from build123d import *

# Parameters (mm, degrees)
SKETCH044_R             = 6.3
SKETCH044_R_2           = 4.2
PAD022_DEPTH            = 0.4
SKETCH049_R             = 5
SKETCH049_R_2           = 4.2
PAD027_DEPTH            = 1.2
PAD037_DEPTH            = 0.2
POLARPATTERN_COUNT      = 6
FILLET002_R             = 0.4
BODY009_PLACEMENT_ANGLE = 153


with BuildPart() as part:
    # Sketch044 → Pad022 (new body)
    with BuildSketch(Plane.XY):
        with Locations((1, 0)):
            Circle(SKETCH044_R)
        Circle(SKETCH044_R_2, mode=Mode.SUBTRACT)
    extrude(amount=PAD022_DEPTH)

    # Sketch049 (on Face4 of Pad022) → Pad027 (join)
    with BuildSketch(Plane.XY.offset(0.4)):
        Circle(SKETCH049_R)
        Circle(SKETCH049_R_2, mode=Mode.SUBTRACT)
    extrude(amount=PAD027_DEPTH)

    # Sketch074 (on Face2 of Pad027) → Pad037 (join)
    with BuildSketch(Plane(origin=(0, 0, 0), x_dir=(1, 0, 0), z_dir=(0, 0, -1))):
        with BuildLine():
            ThreePointArc((3.95, -1.4274102424), (4.2, 0), (3.95, 1.4274102424))
            Line((3.95, 1.4274102424), (3.95, -1.4274102424))
        make_face()
    pad037 = extrude(amount=-PAD037_DEPTH)

    # PolarPattern: Pad037 ×6 about axis
    polarpattern_axis = Axis((0, 0, 0), (0, 0, -1))
    for i in range(1, POLARPATTERN_COUNT):
        add(pad037.rotate(polarpattern_axis, i * 360 / POLARPATTERN_COUNT))

    # Fillet002
    fillet002_edges = [part.edges().sort_by_distance(p)[0] for p in [
        (-4.2, 0, 1.6),
    ]]
    fillet(fillet002_edges, radius=FILLET002_R)


with BuildPart() as part_1:
    # Body009 placement: moved
    add(part.part.moved(Location((0, 0, 4))).rotate(Axis((0, 0, 4), (0, 0, 1)), BODY009_PLACEMENT_ANGLE))


solid = part_1.part
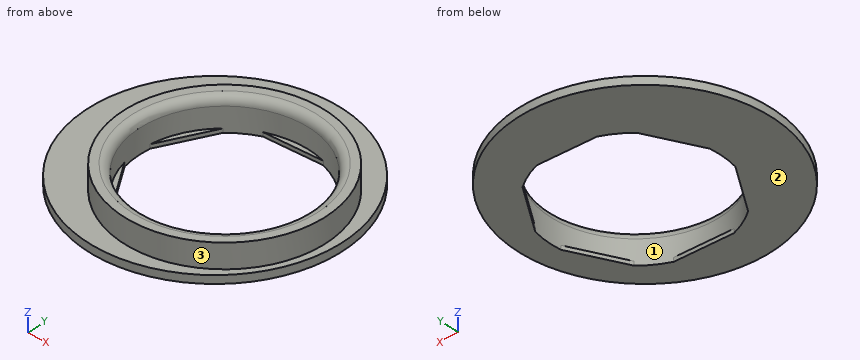
Source: CAD feature listing. Evaluate the final solid. Frame: model axes, mm. Face numbers are marked on the shaded views. Give positions to 0.01 mm unless a question says otherwise; leave off trailing zeros. Write each loop counter-clockwise with the first axis right and the second up, starting at its lowest first coordinate (ties: lowest second). Pieces come first, ordered by that corner, then holes. Notation, with made-up numbers: M 6,-13 L 20,-13 A13 cw 20,0 Z; hole C -14.75,-12 d7. An arc over 180 degrees is marked long. Return JSON: item names as keys, results as strings. Group by question number.
1) Pull-direction query (Y, two-part tool) for the marked faces 1, 2 and 3; classes: pulls with the +Y half, pulls with the -Y half, needs draft (parallel to the pull), parting line crosses it, or undercut.
2) Cut plane C-C, the plane z = 4.55. Output: boundary loops of the cut face in (x, y).
3) Cut plane A-A, the plane x = 0. Output: boundary loops of the cut face in (y, z).
4) Cut plane B-B, the plane y = 0. Output: boundary loops of the cut face in (x, z), plus the area to 3 significant figures.
5) Material intervals for line 1 along Y through (x, z) = (0, 4.55); line 2 along X through (y, z) = (3.75, 5.2); line 3 along Y through (x, z) = (0.5, 4.3), sorted ascending. Write a range as [from, to].
6) Pin query (flat end, axial travel): P1, Ø1, axis at x = -3.5, y = 2, coming from the +Z side. Return the tip coordinate at first contact, or that it passes through.
7) Cut plane D-D, the plane y = 6.25. Output: boundary loops of the cut face in (x, z).
Recorded:
{
 "1": {"face 1": "undercut", "face 2": "needs draft", "face 3": "parting line crosses it"},
 "2": {"outline": "C 0,0 d10; hole C 0,0 d8.4"},
 "3": {"outline": "M -5.78,4 L -3.96,4 L -3.96,4.2 L -4.2,4.2 L -4.2,5.2 A0.4 ccw -4.6,5.6 L -5,5.6 L -5,4.4 L -5.78,4.4 Z; M 3.96,4 L 6.69,4 L 6.69,4.4 L 5,4.4 L 5,5.6 L 4.6,5.6 A0.4 ccw 4.2,5.2 L 4.2,4.2 L 3.96,4.2 Z"},
 "4": {"outline": "M -7.17,4 L -4.2,4 L -4.2,5.2 A0.4 ccw -4.6,5.6 L -5,5.6 L -5,4.4 L -7.17,4.4 Z; M 4.2,4 L 5.39,4 L 5.39,4.4 L 5,4.4 L 5,5.6 L 4.6,5.6 A0.4 ccw 4.2,5.2 Z", "area": "3.52 mm²"},
 "5": {"line 1": "y = [-5, -4.2], [4.2, 5]", "line 2": "x = [-3.31, -1.89], [1.89, 3.31]", "line 3": "y = [-5.69, -4.17], [4.17, 6.6]"},
 "6": {"P1": "stops at z = 5.59"},
 "7": {"outline": "M -3.36,4 L 1.58,4 L 1.58,4.4 L -3.36,4.4 Z"}
}
